```python
from build123d import *

# Parameters (mm, degrees)
SKETCH2_W           = 4
SKETCH2_H           = 15
BOSS_EXTRUDE1_DEPTH = 3


with BuildPart() as part:
    # Sketch1 → Revolve1 (revolve)
    with BuildSketch(Plane(origin=(0, 0, 0), x_dir=(1, 0, 0), z_dir=(0, 1, 0))):
        with BuildLine():
            Line((0, -11.5), (0, 11.5))
            ThreePointArc((0, 11.5), (-11.5, 0), (0, -11.5))
        make_face()
    revolve(axis=Axis((0, 0, 11.5), (0, 0, -1)))

    # Sketch2 → Revolve2 (revolve)
    with BuildSketch(Plane(origin=(0, 0, 0), x_dir=(1, 0, 0), z_dir=(0, 1, 0))):
        with Locations((-2, -17.110144679)):
            Rectangle(SKETCH2_W, SKETCH2_H)
    revolve(axis=Axis((0, 0, 24.610144679), (0, 0, -1)))

    # Sketch3 → Boss-Extrude1 (add)
    with BuildSketch(Plane.XY.offset(9.610144679)):
        Polygon((2.810278521, 4.867545181), (-2.810278521, 4.867545181), (-5.620557041, 0), (-2.810278521, -4.867545181), (2.810278521, -4.867545181), (5.620557041, 0), align=None)
    extrude(amount=BOSS_EXTRUDE1_DEPTH)


solid = part.part
```
Here's how the part is built. I have some questions about the finished solid (model axes, mm). A direction names the side the tool comes from. Coordinates: 2 decimals unless noted, no trailing zeros. Order: outer loops, then holes, each group sorted by start corner. A loop starts at its lowest first (then second) coordinate and runs counter-clockwise, first axis right, second up.
1) Which directions (+Z, -Z, +X, -X, +Y, -Y) give clear straight access to the entire face, cutting with the end or side of a thin tool? Please do faces 1 (the face through (-4.235, -2.4, 11.303)), 2 (the face through (-4.196, 2.468, 11.303)), 3 (the face through (0.867, -3.905, 18.526)).
2) Imagine slicing it at C-C on z = 21. List the corners of the cut face in (x, y) for me.
3) I need wall thicknesses on line 1 (Y direction, x = -5.75, z = 5); line 2 (X direction, y = -0.5, z = 16.5); line 3 (Z direction, x = -9, y = -5.75). Which ranges of each line are inside material? Lowest first, please.
4) Imagine slicing it at D-D on z = -8.5. List the corners of the cut face in (x, y) for me, and give its area (3 significant figures).
5) Imagine slicing it at B-B on y = -1.5. List the corners of the cut face in (x, z) for me, and give its area (3 significant figures).
6) Imagine slicing it at A-A on x = 0. List the corners of the cut face in (y, z) for me, and give its area (3 significant figures).
7) Will these pins go through, and if not, where does the flat tip stop? pin 1 (3 mm diameter, centred on x = -0.5, z = 11, fed in from +Y); pin 2 (5 mm diameter, centred on x = -7.5, z = 3, fed in from +Y); pin 3 (1 mm diameter, centred on x = 8.5, z = 1.5, fed in from +Y).
Response values:
1. face 1: +Z, -X, -Y
1. face 2: +Z, -X, +Y
1. face 3: +Z
2. outline: circle Ø8 at (0, 0)
3. line 1: y = -8.61 to 8.61
3. line 2: x = -3.97 to 3.97
3. line 3: z = -4.26 to 4.26
4. outline: circle Ø15.49 at (0, 0)
4. area: 188 mm2
5. outline: (-4.75, 10.36) arc R11.4 ccw (long way) to (4.75, 10.36) - (4.75, 12.61) - (3.71, 12.61) - (3.71, 24.61) - (-3.71, 24.61) - (-3.71, 12.61) - (-4.75, 12.61) - close
5. area: 512 mm2
6. outline: (-4.87, 10.42) arc R11.5 ccw (long way) to (4.87, 10.42) - (4.87, 12.61) - (4, 12.61) - (4, 24.61) - (-4, 24.61) - (-4, 12.61) - (-4.87, 12.61) - close
6. area: 526 mm2
7. pin 1: stops at y = 6.46
7. pin 2: stops at y = 10.06
7. pin 3: stops at y = 8.13
